Work out the finished part from the listing and answer in its coordinate system (mm). A direction names the side the tool comes from. Give positions to 0.01 mm unless a question says otherwise; leave off trailing zeros. Loops run counter-clockwise (first coordinate to the right, second up) from the corner with the lowest first, then second, coordinate; pieces in that order, holes last. Notation, with made-up numbers: M -34.5,6.5 L 7.5,6.5 A21 cw 7.5,45.5 Z; hole C 20,70 d5. An arc over 180 degrees is marked long. Use a Markdown table: item, result.
```python
from build123d import *

# Parameters (mm, degrees)
SKETCH5_W                 = 11.25
SKETCH5_H                 = 8.5
EXTRUDE4_DEPTH            = 2.5
SKETCH19_W                = 1.5
SKETCH19_H                = 8.5
EXTRUDE12_DEPTH           = 1.5
SKETCH21_W                = 9
SKETCH21_H                = 7
EXTRUDE13_DEPTH           = 3.5
SKETCH22_W                = 4
SKETCH22_H                = 2.5
EXTRUDE14_DEPTH           = 3.75
EXTRUDE15_DEPTH           = 0.75
F_0_80_TAPPED_HOLE1_D     = 1.19126
F_0_80_TAPPED_HOLE1_DEPTH = 79.01
F_0_80_TAPPED_HOLE1_TIP   = 0.357890611
FILLET4_R                 = 1
EXTRUDE16_DEPTH           = 0.75
EXTRUDE17_DEPTH           = 0.75


with BuildPart() as part:
    # Sketch5 → Extrude4 (new body)
    with BuildSketch(Plane(origin=(0, 0, 0), x_dir=(1, 0, 0), z_dir=(0, 1, 0))):
        Rectangle(SKETCH5_W, SKETCH5_H)
    extrude(amount=EXTRUDE4_DEPTH)

    # Sketch19 → Extrude12 (cut)
    with BuildSketch(Plane(origin=(0, 2.5, 0), x_dir=(-1, 0, 0), z_dir=(0, 1, 0))):
        with Locations((4.875, 0)):
            Rectangle(SKETCH19_W, SKETCH19_H)
    extrude(amount=-EXTRUDE12_DEPTH, mode=Mode.SUBTRACT)

    # Sketch21 → Extrude13 (cut, through all)
    with BuildSketch(Plane(origin=(0, 2.5, 0), x_dir=(-1, 0, 0), z_dir=(0, 1, 0))):
        with Locations((-0.375, 0)):
            Rectangle(SKETCH21_W, SKETCH21_H)
    extrude(amount=-EXTRUDE13_DEPTH, mode=Mode.SUBTRACT)

    # Sketch22 → Extrude14 (add)
    with BuildSketch(Plane.XY.offset(4.25)):
        with Locations((-0.875, 1.25)):
            Rectangle(SKETCH22_W, SKETCH22_H)
    extrude(amount=EXTRUDE14_DEPTH)

    # Sketch24 → Extrude15 (add)
    with BuildSketch(Plane(origin=(0, 2.5, 0), x_dir=(1, 0, 0), z_dir=(0, 1, 0))):
        Polygon((-4.125, 3.85), (-4.125, 3.5), (4.875, 3.5), (4.875, -3.5), (-4.125, -3.5), (-4.125, -3.85), (5.225, -3.85), (5.225, 3.85), align=None)
    extrude(amount=EXTRUDE15_DEPTH)

    # #0-80 Tapped Hole1
    with Locations(Plane(origin=(-0.875, 2.5, 6), x_dir=(0, 0, 1), z_dir=(0, 1, 0))):
        with Locations((0, 0)):
            Hole(F_0_80_TAPPED_HOLE1_D / 2, depth=F_0_80_TAPPED_HOLE1_DEPTH)
            with Locations((0, 0, -(F_0_80_TAPPED_HOLE1_DEPTH + F_0_80_TAPPED_HOLE1_TIP / 2))):  # 118° drill point
                Cone(0, F_0_80_TAPPED_HOLE1_D / 2, F_0_80_TAPPED_HOLE1_TIP, mode=Mode.SUBTRACT)

    # Fillet4
    fillet4_edges = [part.edges().sort_by_distance(p)[0] for p in [
        (5.625, 1.25, -4.25),
        (5.225, 2.875, -3.85),
        (5.625, 1.25, 4.25),
        (5.225, 2.875, 3.85),
        (4.875, 1.625, 3.5),
        (4.875, 1.625, -3.5),
        (-4.125, 0.5, 3.5),
        (-4.125, 0.5, -3.5),
        (-5.625, 0.5, -4.25),
        (-5.625, 0.5, 4.25),
        (-2.875, 1.25, 4.25),
        (-2.875, 1.25, 8),
        (1.125, 1.25, 8),
        (1.125, 1.25, 4.25),
    ]]
    fillet(fillet4_edges, radius=FILLET4_R)

    # Sketch28 → Extrude16 (cut)
    with BuildSketch(Plane(origin=(0, 3.25, 0), x_dir=(-1, 0, 0), z_dir=(0, 1, 0))):
        with BuildLine():
            Line((3.125, -3.85), (4.125, -3.85))
            Line((4.125, -3.85), (4.125, -2.85))
            ThreePointArc((4.125, -2.85), (3.832106781, -3.557106781), (3.125, -3.85))
        make_face()
    extrude(amount=-EXTRUDE16_DEPTH, mode=Mode.SUBTRACT)

    # Sketch31 → Extrude17 (cut)
    with BuildSketch(Plane(origin=(0, 3.25, 0), x_dir=(-1, 0, 0), z_dir=(0, 1, 0))):
        with BuildLine():
            Line((4.125, 2.85), (4.125, 3.85))
            Line((4.125, 3.85), (3.125, 3.85))
            ThreePointArc((3.125, 3.85), (3.832106781, 3.557106781), (4.125, 2.85))
        make_face()
    extrude(amount=-EXTRUDE17_DEPTH, mode=Mode.SUBTRACT)


solid = part.part
```
(1) A cutting plane is placed at D-D (y = 1.8). Write down the section's boundary in (x, z) (3 decimals).
Entries:
| item | result |
|---|---|
| outline | M -4.125,-4.25 L 4.625,-4.25 A1 ccw 5.625,-3.25 L 5.625,3.25 A1 ccw 4.625,4.25 L 2.125,4.25 A1 cw 1.125,5.25 L 1.125,7 A1 ccw 0.125,8 L -1.875,8 A1 ccw -2.875,7 L -2.875,5.25 A1 cw -3.875,4.25 L -4.125,4.25 L -4.125,3.5 L 3.875,3.5 A1 cw 4.875,2.5 L 4.875,-2.5 A1 cw 3.875,-3.5 L -4.125,-3.5 Z; hole C -0.875,6 d1.191 |
(2) A cutting plane is placed at A-A (z = 6). Write down the section's boundary in (x, y) (3 decimals), and give its area (3 significant figures).
Entries:
| item | result |
|---|---|
| outline | M -2.875,0 L -1.471,0 L -1.471,2.5 L -2.875,2.5 Z; M -0.279,0 L 1.125,0 L 1.125,2.5 L -0.279,2.5 Z |
| area | 7.02 mm² |
(3) Which of the six approach directions +Z, -Z, +X, -X, +Y, -Y give full straight-line access (tool end or side, diameter ignored) to faces 5 (the flat face through (3, 1, 4.25)), 6 (the cylindrical face through (5.324, 1.268, -3.965)), 7 (the flat face through (5.04, 3.25, -0.02)), 8 (the flat face through (-4.125, 0.5, 0)), 9 (the flat face through (-2.875, 1, 6))?
Entries:
| item | result |
|---|---|
| face 5 | +Z, +X, +Y, -Y |
| face 6 | -Z, +X, +Y, -Y |
| face 7 | +Z, -Z, +X, -X, +Y |
| face 8 | +Y, -Y |
| face 9 | +Z, -X, +Y, -Y |
(4) The mould has two halves that part along Z. Classify faces 1 (the flat face through (0, 1, -4.25)), 2 (the cylindrical face through (4.574, 1.648, -3.215)), 3 (the cylindrical face through (-1.2, 1.2, 6.5)), 4 (the flat face through (-1, 1, 8)): released by +Z, released by -Z, zero draft, split by the parting line, or undercut.
Entries:
| item | result |
|---|---|
| face 1 | released by -Z |
| face 2 | undercut |
| face 3 | undercut |
| face 4 | released by +Z |
(5) A cutting plane is placed at C-C (x = 0.75). Write down the section's boundary in (y, z), and give its area (3 significant figures).
Entries:
| item | result |
|---|---|
| outline | M 0,-4.25 L 2.5,-4.25 L 2.5,-3.85 L 3.25,-3.85 L 3.25,-3.5 L 0,-3.5 Z; M 0,3.5 L 3.25,3.5 L 3.25,3.85 L 2.5,3.85 L 2.5,7.78 L 0,7.78 Z |
| area | 13.1 mm² |
(6) Consider probe 1 along X at (y, z) = (0.85, 6) (3 decimals); probe 2 along Z at (x, y) = (2, 2.65); probe 3 along Z at (x, y) = (2.75, 0.45). Determine where each line is inside the solid, lowest interval first. Write a range as [from, to].
Entries:
| item | result |
|---|---|
| probe 1 | x = [-2.875, -1.471], [-0.279, 1.125] |
| probe 2 | z = [-3.85, -3.5], [3.5, 3.85] |
| probe 3 | z = [-4.25, -3.5], [3.5, 4.25] |
(7) A cutting plane is placed at B-B (y = 0.6). Write down the section's boundary in (x, z) (3 decimals).
Entries:
| item | result |
|---|---|
| outline | M -5.625,-3.25 A1 ccw -4.625,-4.25 L 4.625,-4.25 A1 ccw 5.625,-3.25 L 5.625,3.25 A1 ccw 4.625,4.25 L 2.125,4.25 A1 cw 1.125,5.25 L 1.125,7 A1 ccw 0.125,8 L -1.875,8 A1 ccw -2.875,7 L -2.875,5.25 A1 cw -3.875,4.25 L -4.625,4.25 A1 ccw -5.625,3.25 Z; hole M -4.125,-2.5 A1 ccw -3.125,-3.5 L 3.875,-3.5 A1 ccw 4.875,-2.5 L 4.875,2.5 A1 ccw 3.875,3.5 L -3.125,3.5 A1 ccw -4.125,2.5 Z; hole C -0.875,6 d1.191 |
(8) Given P1, Ø2, axis at x = -4, z = -1, coming from the +Y side; P2, Ø0.5, axis at y = 1, z = 6, coming from the +X side (3 decimals); P3, Ø0.6, axis at y = 2, z = 4, coming from the -X side (3 decimals), each flat-ended and moving along its own axis, determine where each tip first touches the part or whether it passes through.
Entries:
| item | result |
|---|---|
| P1 | stops at y = 1 |
| P2 | stops at x = 1.125 |
| P3 | stops at x = -4.125 |
